Design review of the part shown in the three views and the two pictorial views. Dimensions are in mm from the part's minimum x, y and z. A direction names the side the tool comes from. Coordinates: 2 decimals unless noted, no trailing zeros. Loops run counter-clockwise (first coordinate to the right, second up) from the corner with the lowest first, then second, coordinate; pieces in that order, holes last. Notation, with made-up numbers: M 71.25,75.25 L 99.25,75.25 A21 cw 99.25,103.25 Z; hole C 5.5,-24.5 d7. An arc over 180 degrees is marked long. Answer as a JSON object with one key per item and string values. Group by question number.
Item 1: Add section D-D (x = 13.25). State the section outline as (y, z) points.
Item 2: Add section A-A (x = 7.5). State the section outline as (y, z) points.
Item 3: Insertion check: pin 1 (2 mm diameter, centred on x = 3, z = 5, fed in from +Y); pin 2 (1.5 mm diameter, centred on y = 27.5, z = 10, fed in from +X); pin 3 (1 mm diameter, centred on y = 26, z = 8, fed in from -X). Each pin has a flat end and moves straight along its axis. Give the tip position at first contact, or say it passes through.
Item 4: Add section C-C (y = 17). State the section outline as (x, z) points, then the cut area to 3 significant figures.
Item 5: Add section B-B (z = 7.5). State the section outline as (x, y) points.
Item 6: Tool access review of the marked faces 1 and 2: name each direction out of +Z, -Z, +X, -X, +Y, -Y from which nothing blocks a thin tool from reaching the whole face with its end or side.
Item 7: Wall thickness on L1, parallel to X at y = 8, z = 7.25; L2, parallel to Y at x = 1.5, z = 3.75: over which ranges is each line inside the solid? List them lowest first. Write a range as from..to.
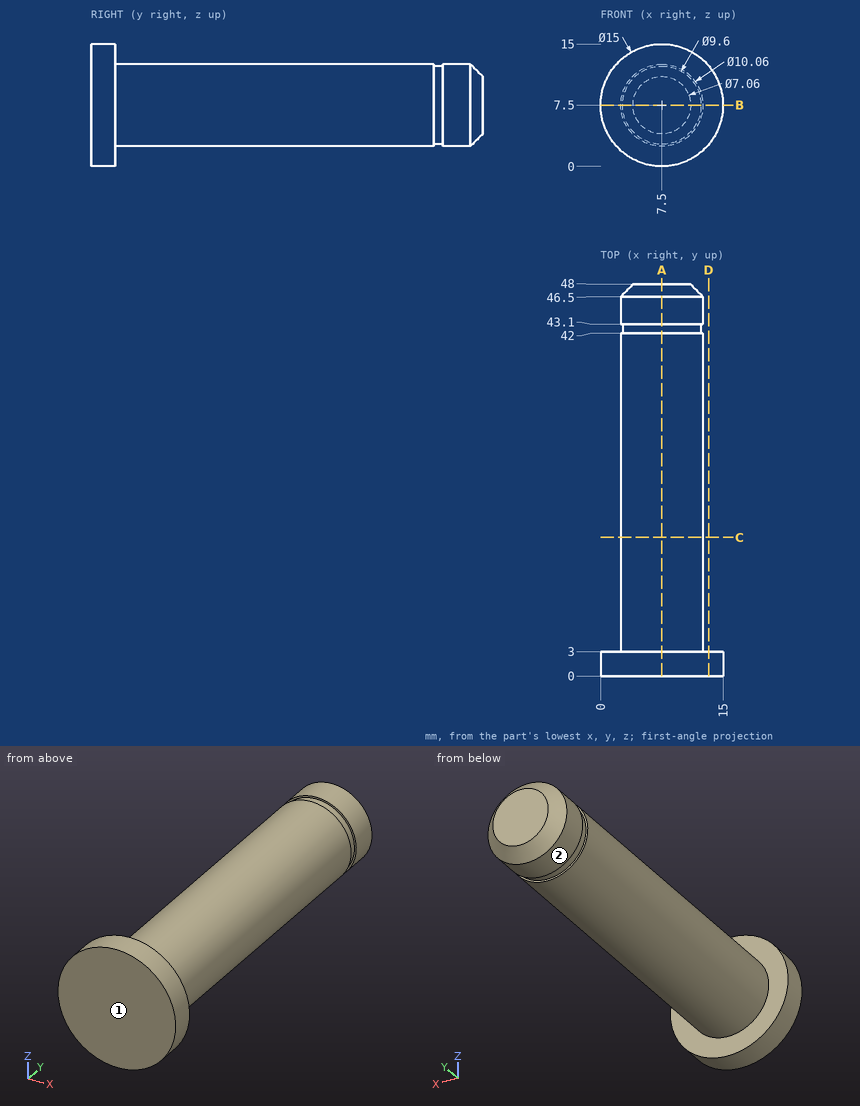
From the geometry:
{
 "1": {"outline": "M 0,2.68 L 3,2.68 L 3,12.32 L 0,12.32 Z"},
 "2": {"outline": "M 0,0 L 3,0 L 3,2.47 L 42,2.47 L 42,2.7 L 43.1,2.7 L 43.1,2.47 L 46.5,2.47 L 48,3.97 L 48,11.03 L 46.5,12.53 L 43.1,12.53 L 43.1,12.3 L 42,12.3 L 42,12.53 L 3,12.53 L 3,15 L 0,15 Z"},
 "3": {"pin 1": "stops at y = 47.38", "pin 2": "stops at x = 12.22", "pin 3": "stops at x = 2.47"},
 "4": {"outline": "C 7.5,7.5 d10.06", "area": "79.5 mm²"},
 "5": {"outline": "M 0,0 L 15,0 L 15,3 L 12.53,3 L 12.53,42 L 12.3,42 L 12.3,43.1 L 12.53,43.1 L 12.53,46.5 L 11.03,48 L 3.97,48 L 2.47,46.5 L 2.47,43.1 L 2.7,43.1 L 2.7,42 L 2.47,42 L 2.47,3 L 0,3 Z"},
 "6": {"face 1": "+Z, -Z, +X, -X, -Y", "face 2": "+Y"},
 "7": {"L1": "x = 2.48..12.52", "L2": "y = 0..3"}
}
